Geometry: final body of the model. Coordinates: model frame, mm. Face numbers are marked on the shaded views. A direction names the side the tool comes from. Round coordinates to 2 decimals unless told otherwise and drop trailing zeros. Loops run counter-clockwise (first coordinate to the right, second up) from the corner with the lowest first, then second, coordinate; pieces in that order, holes last. Notation, with made-up numbers: (-24, 40.25) - (26, 40.25) arc R8 cw to (26, 48.25) - close; hole circle Ø5 at (-18, -22). An arc over 180 degrees is marked (long way). Return JSON: item names as keys, results as strings. Group by question number.
1. Draft query along X for the marked faces 4, 5 and 6. Return one class per face: +X half, -X half, draft (parallel to the pull), parting line (faces both ways), or undercut.
2. Material intervals for probe 1 along X at (y, z) = (12, 18); probe 2 along Y at (x, z) = (73, 27); probe 3 along Z at (x, y) = (90.5, 88), sorted ascending.
3. Section A-A on z = 14.5. Return loops of the section in (x, y), and give its area (3 significant figures).
4. Section C-C on x = 37.5. Return loops of the section in (y, z).
5. Set-up query: the marked faces 1, 2 and 3. Return all of +Z, -Z, +X, -X, +Y, -Y with unobstructed straight access to the full face (end or side cutting, diameter ignored); none if empty.
6. Section B-B on y = 61.5. Return loops of the section in (x, z), and give its area (3 significant figures).
7. First-contact query: pin 1 Ø8 at (x, y) = (53.5, 75) entering from -Z; pin 2 Ø2.5 at (y, z) = (54.5, -3) entering from -X. Flat tips, straight axial feed; report the tip coordinate or a pass-through.
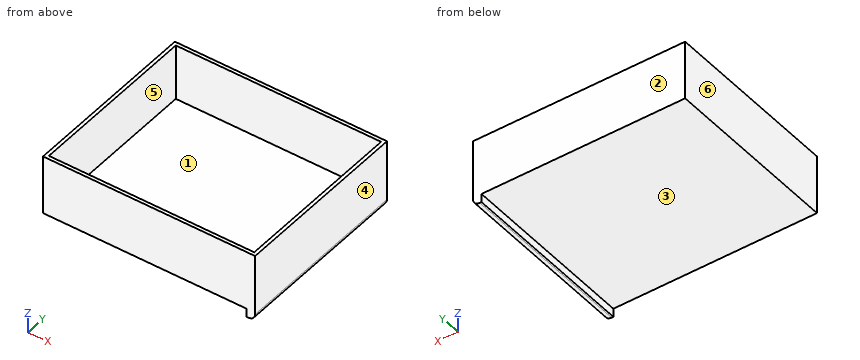
from build123d import *

# Parameters (mm, degrees)
SKETCH_1_W      = 125
SKETCH_1_H      = 105.8
EXTRUDE_1_DEPTH = 35
SHELL_1_T       = -2
SKETCH_2_W      = 5
SKETCH_2_H      = 105.8
EXTRUDE_2_DEPTH = 5
FILLET_1_R      = 4


with BuildPart() as part:
    # 草图1 → 凸台-拉伸1 (new body)
    with BuildSketch(Plane.XY):
        with Locations((62.5, 52.9)):
            Rectangle(SKETCH_1_W, SKETCH_1_H)
    extrude(amount=EXTRUDE_1_DEPTH)

    # 抽壳1
    shell_1_openings = [part.faces().sort_by_distance(p)[0] for p in [
        (62.5, 52.9, 35),
    ]]
    offset(amount=SHELL_1_T, openings=shell_1_openings, kind=Kind.INTERSECTION)

    # 草图2 → 凸台-拉伸2 (add)
    with BuildSketch(Plane(origin=(0, 0, 0), x_dir=(-1, 0, 0), z_dir=(0, 0, -1))):
        with Locations((-122.5, 52.9)):
            Rectangle(SKETCH_2_W, SKETCH_2_H)
    extrude(amount=EXTRUDE_2_DEPTH)

    # 圆角1
    fillet_1_edges = [part.edges().sort_by_distance(p)[0] for p in [
        (125, 52.9, -5),
    ]]
    fillet(fillet_1_edges, radius=FILLET_1_R)


solid = part.part
Taken from the geometry:
{
 "1": {"face 4": "+X half", "face 5": "undercut", "face 6": "-X half"},
 "2": {"probe 1": "0 to 2, 123 to 125", "probe 2": "0 to 2, 103.8 to 105.8", "probe 3": "0 to 2"},
 "3": {"outline": "(0, 0) - (125, 0) - (125, 105.8) - (0, 105.8) - close; hole (2, 2) - (123, 2) - (123, 103.8) - (2, 103.8) - close", "area": "907 mm2"},
 "4": {"outline": "(0, 0) - (105.8, 0) - (105.8, 35) - (103.8, 35) - (103.8, 2) - (2, 2) - (2, 35) - (0, 35) - close"},
 "5": {"face 1": "+Z", "face 2": "+Z, -Z, +X, -X, +Y", "face 3": "-Z, -X, +Y, -Y"},
 "6": {"outline": "(0, 0) - (120, 0) - (120, -5) - (121, -5) arc R4 ccw to (125, -1) - (125, 35) - (123, 35) - (123, 2) - (2, 2) - (2, 35) - (0, 35) - close", "area": "404 mm2"},
 "7": {"pin 1": "z = 0", "pin 2": "x = 120"}
}
